Geometry: final body of the model. Coordinates: model frame, mm. Face numbers are marked on the shaded views. A direction names the side the tool comes from. Give positions to 0.01 mm unless a question says otherwise; leave off trailing zeros. Loops run counter-clockwise (first coordinate to the right, second up) from the corner with the lowest first, then second, coordinate; pieces in that order, holes last.
1. Section A-A, the plane z = -34. Output: boundary loops of the cut face in (x, y).
2. Material intervals for line 1 along Z through (x, y) = (0, 2); line 2 along Z through (x, y) = (3.5, -9.5); line 3 along X through (y, z) = (7.5, -39), sorted ascending.
3. Section B-B, the plane y = 7. State how many separate pieces and enclosed holes the cut face has, then the cut area to 3 significant figures.
4. First-contact query: P1, Ø1.5, axis at y = 0.5, z = -45, coming from the -X side; P2, Ø12, axis at x = 13, y = 8.5, coming from the +Z side (3 decimals); P3, Ø3, axis at x = -0.5, y = 14.5, coming from the +Z side; P4, Ø19, axis at x = 0, z = 40, coming from the -Y side. Flat tips, straight axial feed; report the tip coordinate or a pass-through.
5. Section C-C, the plane x = -7. Output: boundary loops of the cut face in (y, z) (3 decimals).
6. Section D-D, the plane z = 44.5. Output: boundary loops of the cut face in (x, y).
7. Access query for the marked faces 1, 2 and 3. Directions: +Z, -Z, +X, -X, +Y, -Y. A direction counts if a zero-diameter tool reaches every point of the face in a straight line with its end or side. Return the directions, or none.
8. Draft query along Z for the marked faces 4, 5, 6 and 7. Return one class per face: +Z half, -Z half, draft (parallel to the pull), parting line (faces both ways), or undercut.
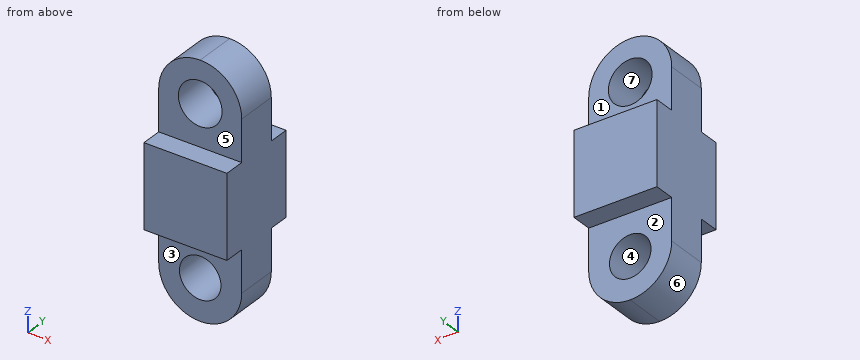
from build123d import *

# Parameters (mm, degrees)
F0_W     = 40
F0_H     = 120
F1_DEPTH = 10
F2_W     = 40
F2_H     = 40
F3_DEPTH = 10
F5_R     = 10.5368442401
F6_DEPTH = 20
F7_R     = 10
F8_DEPTH = 20
F9_R     = 19.99999
F10_R    = 19.99999


# Not quite as in the source:
# - a fillet or chamfer is up to 0.001 mm smaller than in the source, because OpenCascade refuses the exact size


with BuildPart() as f1:
    # F0 (on Front) → F1 (new body)
    with BuildSketch(Plane.XZ):
        Rectangle(F0_W, F0_H)
    extrude(amount=F1_DEPTH)

    # F2 (on face) → F3 (join)
    with BuildSketch(Plane.XZ.offset(10)):
        Rectangle(F2_W, F2_H)
    extrude(amount=F3_DEPTH)

    # F4: F1 across face


with BuildPart() as f1_1:
    add(f1.part)
    add(f1.part.mirror(Plane(origin=(0, 0, 0), x_dir=(1, 0, 0), z_dir=(0, 1, 0))))

    # F5 (on face) → F6 (cut, through all)
    with BuildSketch(Plane.XZ.offset(10)):
        with Locations((0, 40)):
            Circle(F5_R)
    extrude(amount=-F6_DEPTH, mode=Mode.SUBTRACT)

    # F7 (on face) → F8 (cut, through all)
    with BuildSketch(Plane(origin=(0, 10, 0), x_dir=(-1, 0, 0), z_dir=(0, 1, 0))):
        with Locations((0, -40)):
            Circle(F7_R)
    extrude(amount=-F8_DEPTH, mode=Mode.SUBTRACT)

    # F9 (radius 20 in the source; OpenCascade refuses exactly that, so slightly less here)
    f9_edges = [f1_1.edges().sort_by_distance(p)[0] for p in [
        (-20, 0, 60),
        (20, 0, 60),
    ]]
    fillet(f9_edges, radius=F9_R)

    # F10 (radius 20 in the source; OpenCascade refuses exactly that, so slightly less here)
    f10_edges = [f1_1.edges().sort_by_distance(p)[0] for p in [
        (20, 0, -60),
        (-20, 0, -60),
    ]]
    fillet(f10_edges, radius=F10_R)


solid = f1_1.part
Answers below:
1. outline: (-20, -10) - (-8, -10) - (-8, 10) - (-20, 10) - close; (8, -10) - (20, -10) - (20, 10) - (8, 10) - close
2. line 1: z = -60 to -50, -30 to 29.46, 50.54 to 60
2. line 2: z = -59.69 to -49.37, -30.63 to 30.06, 49.94 to 59.69
2. line 3: x = -20 to -9.95, 9.95 to 20
3. separate pieces: 1
3. enclosed holes: 2
3. area: 3,790 mm2
4. P1: stops at x = -19.54
4. P2: stops at z = 58.735
4. P3: stops at z = 20
4. P4: passes through
5. outline: (-20, -20) - (-10, -20) - (-10, -32.859) - (10, -32.859) - (10, -20) - (20, -20) - (20, 20) - (10, 20) - (10, 32.124) - (-10, 32.124) - (-10, 20) - (-20, 20) - close; (-10, -58.735) - (10, -58.735) - (10, -47.141) - (-10, -47.141) - close; (-10, 47.876) - (10, 47.876) - (10, 58.735) - (-10, 58.735) - close
6. outline: (-19.49, -10) - (-9.53, -10) - (-9.53, 10) - (-19.49, 10) - close; (9.53, -10) - (19.49, -10) - (19.49, 10) - (9.53, 10) - close
7. face 1: +Z, +X, -X, +Y
7. face 2: -Z, +X, -X, +Y
7. face 3: -Z, +X, -X, -Y
8. face 4: undercut
8. face 5: draft
8. face 6: -Z half
8. face 7: undercut
